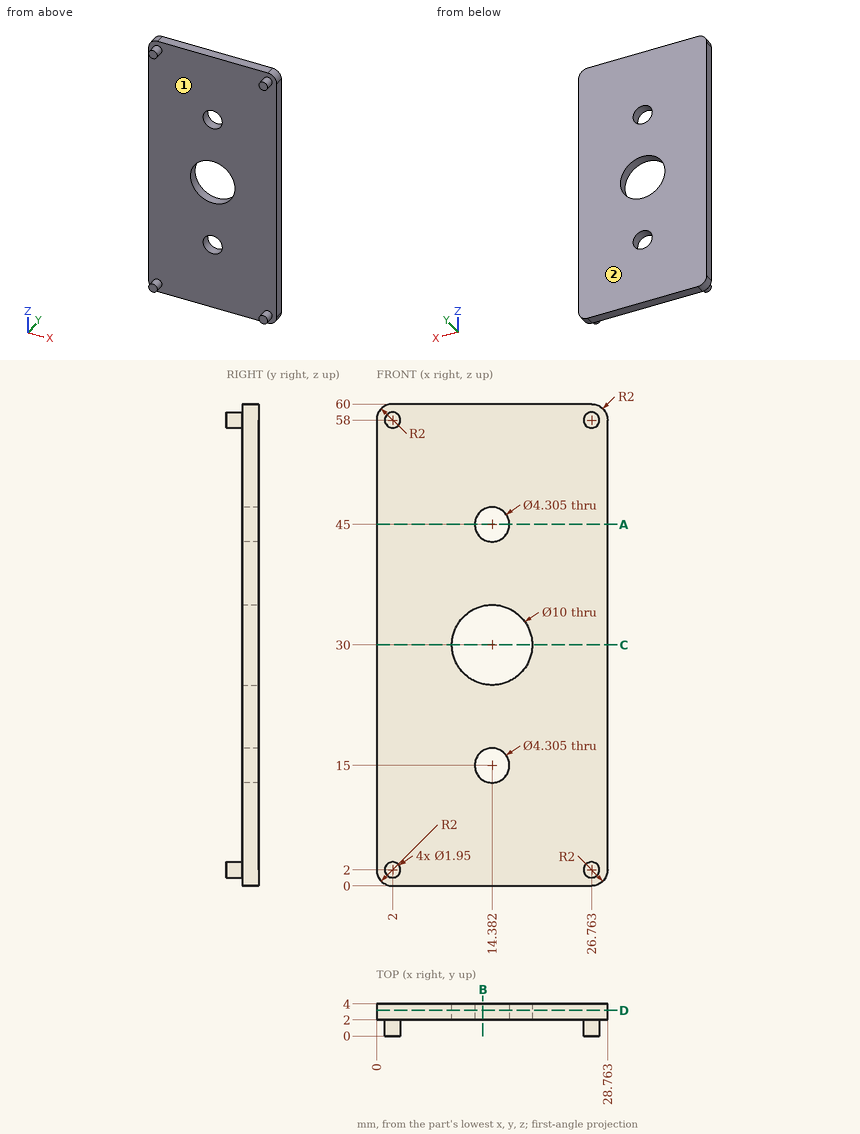
Could you check a few things on this drawing? It's one solid part, dimensions in mm from its lowest x, y, z. Coordinates: 2 decimals unless noted, no trailing zeros. Order: outer loops, then holes, each group sorted by start corner. A loop starts at its lowest first (then second) coordinate and runs counter-clockwise, first axis right, second up.
1) I need wall thicknesses on line 1 (X direction, y = 3.55, z = 30); line 2 (Z direction, x = 12.75, y = 2.85) (1 decimal); line 3 (X direction, y = 3.35, z = 45) (1 decimal). Which ranges of each line are inside material? Lowest first, please.
2) Imagine slicing it at D-D on y = 3.2. List the corners of the cut face in (x, z) for me (1 decimal).
3) Imagine slicing it at C-C on z = 30. List the corners of the cut face in (x, y) for me.
4) Imagine slicing it at B-B on x = 13.25. List the corners of the cut face in (y, z) for me.
5) Imagine slicing it at A-A on z = 45. List the corners of the cut face in (x, y) for me (1 decimal).
6) Will this pin go through, and if not, where does the flat tip stop? pin 1 (10 mm diameter, centred on x = 3.5, z = 23.5, fed in from -Y).
7) We'd pull the mould along Z, two halves only. Please class the marked faces 1 and 2: +Z half, -Z half, draft (parallel to the pull), parting line (faces both ways), or undercut.
Response values:
1. line 1: x = 0 to 9.38, 19.38 to 28.76
1. line 2: z = 0 to 13.6, 16.4 to 25.3, 34.7 to 43.6, 46.4 to 60
1. line 3: x = 0 to 12.2, 16.5 to 28.8
2. outline: (0, 2) arc R2 ccw to (2, 0) - (26.8, 0) arc R2 ccw to (28.8, 2) - (28.8, 58) arc R2 ccw to (26.8, 60) - (2, 60) arc R2 ccw to (0, 58) - close; hole circle Ø10 at (14.4, 30); hole circle Ø4.3 at (14.4, 15); hole circle Ø4.3 at (14.4, 45)
3. outline: (0, 2) - (9.38, 2) - (9.38, 4) - (0, 4) - close; (19.38, 2) - (28.76, 2) - (28.76, 4) - (19.38, 4) - close
4. outline: (2, 0) - (4, 0) - (4, 13.17) - (2, 13.17) - close; (2, 16.83) - (4, 16.83) - (4, 25.13) - (2, 25.13) - close; (2, 34.87) - (4, 34.87) - (4, 43.17) - (2, 43.17) - close; (2, 46.83) - (4, 46.83) - (4, 60) - (2, 60) - close
5. outline: (0, 2) - (12.2, 2) - (12.2, 4) - (0, 4) - close; (16.5, 2) - (28.8, 2) - (28.8, 4) - (16.5, 4) - close
6. pin 1: stops at y = 2
7. face 1: undercut
7. face 2: draft
